from build123d import *

# Parameters (mm, degrees)
F0_W     = 3
F0_H     = 20
F1_DEPTH = 15
F3_D     = 4.5
F3_DEPTH = 4
F3_TIP   = 1.3519363928
F5_D     = 4.5
F6_R     = 7.5
F7_R     = 7.49999


# Not quite as in the source:
# - a fillet or chamfer is up to 0.001 mm smaller than in the source, because OpenCascade refuses the exact size


with BuildPart() as f1:
    # F0 (on Front) → F1 (new body)
    with BuildSketch(Plane.XZ):
        with Locations((25.3187853247, -10)):
            Rectangle(F0_W, F0_H)
        with Locations((48.3187853247, -10)):
            Rectangle(F0_W, F0_H)
        Polygon((49.8187853247, 3), (-80.1812146753, 3), (-80.1812146753, 0), (23.8187853247, 0), (26.8187853247, 0), (46.8187853247, 0), (49.8187853247, 0), align=None)
    extrude(amount=F1_DEPTH)

    # F3
    with Locations(Plane(origin=(0, 0, 0), x_dir=(1, 0, 0), z_dir=(0, 0, -1))):
        with Locations((-72.5346971303, 7.5479238294)):
            Hole(F3_D / 2, depth=F3_DEPTH)
            with Locations((0, 0, -(F3_DEPTH + F3_TIP / 2))):  # 118° drill point
                Cone(0, F3_D / 2, F3_TIP, mode=Mode.SUBTRACT)

    # F5 (through all)
    with Locations(Plane.YZ.offset(49.8187853247)):
        with Locations((-7.5, -12.5)):
            Hole(F5_D / 2)

    # F6
    f6_edges = [f1.edges().sort_by_distance(p)[0] for p in [
        (48.318785, 0, -20),
    ]]
    fillet(f6_edges, radius=F6_R)

    # F7 (radius 7.5 in the source; OpenCascade refuses exactly that, so slightly less here)
    f7_edges = [f1.edges().sort_by_distance(p)[0] for p in [
        (25.318785, -15, -20),
        (48.318785, -15, -20),
        (25.318785, 0, -20),
        (-80.181215, 0, 1.5),
        (-80.181215, -15, 1.5),
    ]]
    fillet(f7_edges, radius=F7_R)


solid = f1.part
Here's how the part is built. I have some questions about the finished solid (model axes, mm). A direction names the side the tool comes from. Give positions to 0.01 mm unless a question says otherwise; leave off trailing zeros. Order: outer loops, then holes, each group sorted by start corner. A loop starts at its lowest first (then second) coordinate and runs counter-clockwise, first axis right, second up. Notation, with made-up numbers: M 66,-18 L 84,-18 A15 ccw 84,-3 Z; hole C 59.25,34.5 d10. An arc over 180 degrees is marked long. Answer as a JSON object with one key per item and string values. Group by question number.
1) I'm going to push flat-ended pins straight in: pin 1 Ø2.5 at (y, z) = (-7.5, -12.5) entering from -X; pin 2 Ø7.5 at (x, y) = (39.5, -5.5) entering from -Z; pin 3 Ø7.5 at (y, z) = (-7.5, -8.5) entering from -X. Where does each tip first touch, or does it pass through?
2) Suppose I cut it at D-D, the plane y = -1.25. Write out the boundary of the cut face in (x, z), plus the area to 3 significant figures.
3) Suppose I cut it at A-A, the plane z = -2. Write out the boundary of the cut face in (x, y).
4) Suppose I cut it at C-C, the plane x = 39.5. Write out the boundary of the cut face in (y, z).
5) We'd pull the mould along Z, two halves only. Please class faces 1 (the flat face through (23.819, -7, -10)), 2 (the cylindrical face through (25.34, -12.745, -17.861)), 3 (the cylindrical face through (48.3, -7.21, -10.27)): pulls with the +Z half, pulls with the -Z half, needs draft (parallel to the pull), parting line crosses it, or undercut.
6) On a 3-axis mill with a long thin cutter (end or side, diameter ignored), from which of +Z, -Z, +X, -X, +Y, -Y can I reach the whole of each face in a straight line? I mean faces 4 (the flat face through (-14, -7, 3)), 5 (the flat face through (-29, -7, 0)), 6 (the flat face through (37, -7, 0)). Say none if no direction works.
7) Suppose I cut it at B-B, the plane y = -13. Write out the boundary of the cut face in (x, z), plus the area to 3 significant figures.
8) Please list where these lines run through material, in increasing order: L1, parallel to X at y = -13.75, z = -15.25; L2, parallel to Z at x = 28.5, y = -10; L3, parallel to X at y = -5.75, z = 1. Write a range as [from, to].
Results found:
{
 "1": {"pin 1": "through", "pin 2": "z = 0", "pin 3": "x = 23.82"},
 "2": {"outline": "M -76.83,0 L 23.82,0 L 23.82,-16.65 L 26.82,-16.65 L 26.82,0 L 46.82,0 L 46.82,-16.65 L 49.82,-16.65 L 49.82,3 L -76.83,3 Z", "area": "480 mm²"},
 "3": {"outline": "M 23.82,-15 L 26.82,-15 L 26.82,0 L 23.82,0 Z; M 46.82,-15 L 49.82,-15 L 49.82,0 L 46.82,0 Z"},
 "4": {"outline": "M -15,0 L 0,0 L 0,3 L -15,3 Z"},
 "5": {"face 1": "needs draft", "face 2": "pulls with the -Z half", "face 3": "undercut"},
 "6": {"face 4": "+Z, +X, -X, +Y, -Y", "face 5": "-Z, -X, +Y, -Y", "face 6": "-Z, +Y, -Y"},
 "7": {"outline": "M -77.78,0 L 23.82,0 L 23.82,-17.6 L 26.82,-17.6 L 26.82,0 L 46.82,0 L 46.82,-17.6 L 49.82,-17.6 L 49.82,3 L -77.78,3 Z", "area": "488 mm²"},
 "8": {"L1": "[23.82, 26.82], [46.82, 49.82]", "L2": "[0, 3]", "L3": "[-79.97, -73.89], [-71.18, 49.82]"}
}
